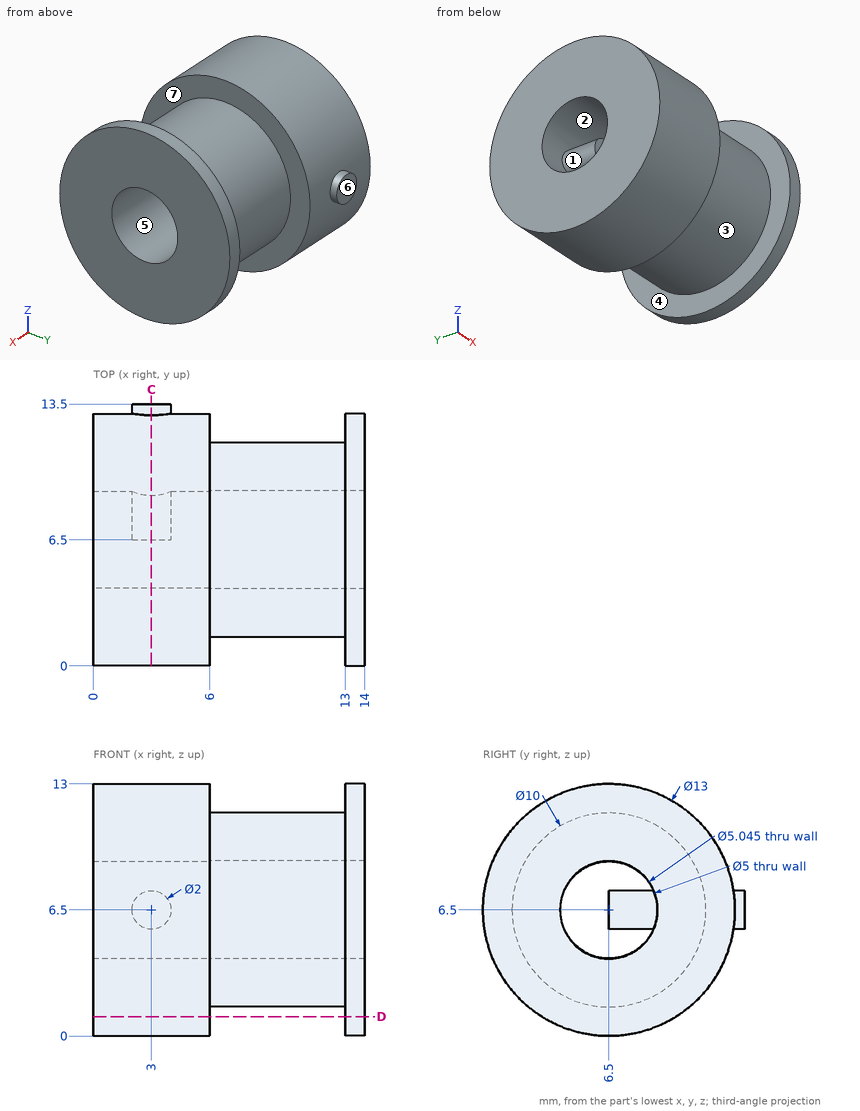
For this review, use the dimensioned drawing (mm, ordinates from the lowest corner) and the shaded views. A direction names the side the tool comes from. Give positions to 0.01 mm unless a question says otherwise; leave off trailing zeros. Order: outer loops, then holes, each group sorted by start corner. A loop starts at its lowest first (then second) coordinate and runs counter-clockwise, first axis right, second up. Notation, with made-up numbers: M 49.5,-2.75 L 103.5,-2.75 A18 cw 103.5,10.25 Z; hole C -7,27 d10. An arc over 180 degrees is marked long. Use one line per item in the form item = value. Start each with the question number.
Item 1: For the marked faces 5, 6 and 7, list the 3-axis set-ups (+Z, -Z, +X, -X, +Y, -Y) from which the entire face can be reached by the end or side of a thin tool; tool diameter is ignored.
Item 2: We need section C-C on x = 3. Give the boundary of the cut face in (y, z).
Item 3: Insertion check: pin 1 Ø4 at (x, y) = (4, 3.5) entering from -Z; pin 2 Ø3 at (x, z) = (9.5, 7) entering from -Y; pin 3 Ø1.5 at (y, z) = (7, 7.5) entering from +X. Each pin has a flat end and moves straight along its axis. Give the tip position at first contact, or say it passes through.
Item 4: The part is to be moulded in two halves that separate along Z. For the marked faces 1, 2, 3 and 4, say which applies: pulls with the +Z half, pulls with the -Z half, needs draft (parallel to the pull), parting line crosses it, or undercut.
Item 5: To check wall thickness, follow line 1 along Z through (x, y) = (9.25, 6.5); line 2 along Z through (x, y) = (2.5, 8.25) (1 decimal); line 3 along X through (y, z) = (1.75, 10). State the ranges of each line that lie inside material, in increasing order. Write a range as from..to.
Item 6: We need section D-D on z = 1. Give the boundary of the cut face in (x, y), plus the area to 3 significant figures.
Completed:
q1.face_5 = +X
q1.face_6 = +Z, -Z, +X, -X, +Y
q1.face_7 = none
q2.outline = M 12.92,5.5 L 13.5,5.5 L 13.5,7.5 L 12.92,7.5 A6.5 ccw long Z; hole M 6.5,5.5 L 6.5,7.5 L 8.79,7.5 A2.5 ccw long 8.79,5.5 Z
q3.pin_1 = 0.08
q3.pin_2 = 1.5
q3.pin_3 = 3.97
q4.face_1 = undercut
q4.face_2 = undercut
q4.face_3 = parting line crosses it
q4.face_4 = needs draft
q5.line_1 = 1.5..3.98, 9.02..11.5
q5.line_2 = 0.2..4.7, 5.6..7.4, 8.3..12.8
q5.line_3 = 0..6, 13..14
q6.outline = M 0,3.04 L 6,3.04 L 6,9.96 L 0,9.96 Z; M 13,3.04 L 14,3.04 L 14,9.96 L 13,9.96 Z
q6.area = 48.5 mm²
